from build123d import *

# Parameters (mm, degrees)
F1_DEPTH      = 42
F1_DEPTH_BACK = 42
F2_DEPTH      = 25
F4_DEPTH      = 65.4
F5_START      = -31.4
F3_W          = 58
F3_H          = 58
F5_DEPTH      = 75.6
F6_START      = -25
F3_W_2        = 2.2413287042
F6_DEPTH      = 53


with BuildPart() as f1:
    # F0 (on Front) → F1 (new body, two sides)
    with BuildSketch(Plane.XZ) as f1_sk:
        Polygon((-31.2413287042, -43), (31.2413287042, -43), (50.5495316972, 16.4245384838), (45.1621487729, 20.3387012929), (39.7747658486, 24.252864102), (29, 32.0811897203), (29, 29), (29, -29), (-29, -29), (-29, 29), (-29, 32.0811897203), (-45.1621487729, 20.3387012929), (-50.5495316972, 16.4245384838), align=None)
        Polygon((39.7747658486, 24.252864102), (45.1621487729, 20.3387012929), (34.6653007859, 47.7126932694), (7.25, 47.8834897045), (14.5, 42.6160563764), (29, 32.0811897203), align=None)
        Polygon((-34.6653007859, 47.7126932694), (-45.1621487729, 20.3387012929), (-29, 32.0811897203), (-7.25, 47.8834897045), align=None)
        Polygon((-7.25, 47.8834897045), (-29, 32.0811897203), (29, 32.0811897203), (14.5, 42.6160563764), (7.25, 47.8834897045), (0, 53.1509230325), align=None)
    extrude(amount=-F1_DEPTH)
    extrude(f1_sk.sketch, amount=F1_DEPTH_BACK)

    # F0 (on Front) → F2 (join)
    with BuildSketch(Plane.XZ):
        Polygon((-31.2413287042, -43), (31.2413287042, -43), (50.5495316972, 16.4245384838), (45.1621487729, 20.3387012929), (39.7747658486, 24.252864102), (29, 32.0811897203), (29, 29), (29, -29), (-29, -29), (-29, 29), (-29, 32.0811897203), (-45.1621487729, 20.3387012929), (-50.5495316972, 16.4245384838), align=None)
        Polygon((39.7747658486, 24.252864102), (45.1621487729, 20.3387012929), (34.6653007859, 47.7126932694), (7.25, 47.8834897045), (14.5, 42.6160563764), (29, 32.0811897203), align=None)
        Polygon((-34.6653007859, 47.7126932694), (-45.1621487729, 20.3387012929), (-29, 32.0811897203), (-7.25, 47.8834897045), align=None)
        Polygon((-7.25, 47.8834897045), (-29, 32.0811897203), (29, 32.0811897203), (14.5, 42.6160563764), (7.25, 47.8834897045), (0, 53.1509230325), align=None)
    extrude(amount=F2_DEPTH)

    # F0 (on Front) → F4 (cut)
    with BuildSketch(Plane.XZ):
        Polygon((-7.25, 47.8834897045), (-29, 32.0811897203), (29, 32.0811897203), (14.5, 42.6160563764), (7.25, 47.8834897045), (0, 53.1509230325), align=None)
    extrude(amount=-F4_DEPTH, mode=Mode.SUBTRACT)

    # F3 (on face) → F5 (cut)
    with BuildSketch(Plane(origin=(0, 0, -43), x_dir=(1, 0, 0), z_dir=(0, 0, -1)).offset(F5_START)):
        Rectangle(F3_W, F3_H)
    extrude(amount=-F5_DEPTH, mode=Mode.SUBTRACT)

    # F3 (on face) → F6 (join)
    with BuildSketch(Plane(origin=(0, 0, -43), x_dir=(1, 0, 0), z_dir=(0, 0, -1)).offset(F6_START)):
        with Locations((-30.1206643521, 0)):
            Rectangle(F3_W_2, F3_H)
        with Locations((30.1206643521, 0)):
            Rectangle(F3_W_2, F3_H)
    extrude(amount=-F6_DEPTH)


solid = f1.part
The listing builds one solid part. Answer for the finished solid, in the listing's coordinates (mm). A direction names the side the tool comes from. Give positions to 0.01 mm unless a question says otherwise; leave off trailing zeros. Write each loop counter-clockwise with the first axis right and the second up, starting at its lowest first coordinate (ties: lowest second). Pieces come first, ordered by that corner, then holes. Notation, with made-up numbers: (77.5, 74.5) - (106.5, 74.5) arc R28 ccw to (106.5, 102.5) - close; hole circle Ø8 at (23.25, -0.5). An arc over 180 degrees is marked (long way). Use a Markdown table: item, result.
1. A tool of negligible diameter and unlimited length cuts with its end or side. For faces 4 (the flat face through (23, 29, 43)), 5 (the flat face through (-29, 1, 9)), 6 (the flat face through (0, -35, 32.081)), from which of +Z, -Z, +X, -X, +Y, -Y can it reach the whole face along a straight path? Write none if from no direction.
Values follow:
| item | result |
|---|---|
| face 4 | +Z |
| face 5 | none |
| face 6 | +Y, -Y |
2. For a pull along X with two mould halves and no side action, classify faces 1 (the flat face through (-17.973, 35.409, 40.093)), 2 (the flat face through (-41.03, 0.59, -12.87)), 3 (the flat face through (47.894, 0.588, 18.354)) as released by +X, released by -X, zero draft, split by the parting line, or undercut.
Values follow:
| item | result |
|---|---|
| face 1 | undercut |
| face 2 | released by -X |
| face 3 | released by +X |
3. Find the intervals of material crossed by probe 1 along Z at (x, y) = (-9, -29.5); probe 2 along Z at (x, y) = (28.5, 25.5); probe 3 along Y at (x, z) = (-13.5, 46.5), in increasing order. Write a range as from..to.
Values follow:
| item | result |
|---|---|
| probe 1 | z = -43..-29, 32.08..47.87 |
| probe 2 | z = -43..-29 |
| probe 3 | y = -42..-29, 29..42 |
4. Section D-D on y = -9 is taken. Write down the section's boundary in (x, z), plus the area to 3 significant figures.
Values follow:
| item | result |
|---|---|
| outline | (-50.55, 16.42) - (-31.24, -43) - (31.24, -43) - (50.55, 16.42) - (45.16, 20.34) - (34.67, 47.71) - (29, 47.75) - (29, -29) - (-29, -29) - (-29, 47.75) - (-34.67, 47.71) - (-45.16, 20.34) - close |
| area | 2,970 mm² |
5. Section A-A on x = 23.5 is taken. Write down the section's boundary in (y, z), plus the area to 3 significant figures.
Values follow:
| item | result |
|---|---|
| outline | (-42, -43) - (42, -43) - (42, -29) - (-42, -29) - close; (-42, 32.08) - (-29, 32.08) - (-29, 47.78) - (-42, 47.78) - close; (29, 36.08) - (42, 36.08) - (42, 47.78) - (29, 47.78) - close |
| area | 1,530 mm² |
6. Section B-B on y = -35 is taken. Write down the section's boundary in (x, z), plus the area to 3 significant figures.
Values follow:
| item | result |
|---|---|
| outline | (-50.55, 16.42) - (-31.24, -43) - (31.24, -43) - (50.55, 16.42) - (45.16, 20.34) - (34.67, 47.71) - (7.25, 47.88) - (0, 53.15) - (-7.25, 47.88) - (-34.67, 47.71) - (-45.16, 20.34) - close; hole (-29, -29) - (29, -29) - (29, 32.08) - (-29, 32.08) - close |
| area | 3,920 mm² |
7. Each of these flat-tipped pins is pushed along its axis until it touches: P1, Ø10, axis at x = 39.5, y = -8.5, coming from the +Z side; P2, Ø1, axis at x = -1.5, y = -1, coming from the +Z side; P3, Ø4, axis at y = -25, z = 1.5, coming from the +X side. Where does it stop, or does it pass through?
Values follow:
| item | result |
|---|---|
| P1 | stops at z = 47.71 |
| P2 | stops at z = -29 |
| P3 | stops at x = 46.35 |
8. Section C-C on z = -20.5 is taken. Write down the section's boundary in (x, y).
Values follow:
| item | result |
|---|---|
| outline | (-38.55, -42) - (-29, -42) - (-29, 42) - (-38.55, 42) - close; (29, -42) - (38.55, -42) - (38.55, 42) - (29, 42) - close |
